Read the model definition and answer for the solid it produces. Units are mm, in the model's axes. Give positions to 0.01 mm unless a question says otherwise; leave off trailing zeros. Write each loop counter-clockwise with the first axis right and the second up, starting at its lowest first coordinate (ties: lowest second). Pieces come first, ordered by that corner, then holes. Notation, with made-up numbers: M 76.5,-9.75 L 107.5,-9.75 A19 cw 107.5,11.25 Z; hole C 17.5,42.5 d5. An arc over 180 degrees is marked long. Put each result on its own line as item: value.
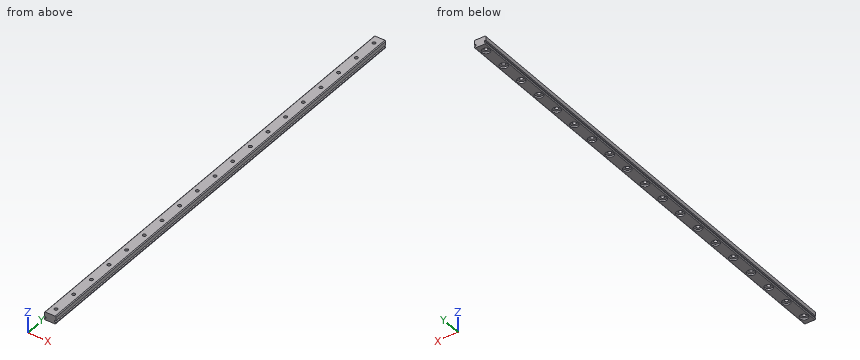
from build123d import *

# Parameters (mm, degrees)
EXTRUDE_1_DEPTH     = 280
SKETCH_2_R          = 1
CUT_EXTRUDE_1_DEPTH = 10
CHAMFER_1_SIZE      = 0.5
SKETCH_3_R          = 2.383304988
CUT_EXTRUDE_2_DEPTH = 1


with BuildPart() as part:
    # 草图1 → 凸台-拉伸1 (new body)
    with BuildSketch(Plane(origin=(0, 0, 0), x_dir=(1, 0, 0), z_dir=(0, 1, 0))):
        Polygon((-3.5, 0.4), (-3.5, -2.4), (3.5, -2.4), (3.5, 0.4), (2.5, 0.4), (2.5, 1.4), (3.5, 1.4), (3.5, 2.4), (-3.5, 2.4), (-3.5, 1.4), (-2.5, 1.4), (-2.5, 0.4), align=None)
    extrude(amount=EXTRUDE_1_DEPTH)

    # 草图2 → 切除-拉伸1 (cut)
    with BuildSketch(Plane(origin=(0, 0, -2.4), x_dir=(-1, 0, 0), z_dir=(0, 0, -1))):
        with Locations((0, 5)):
            Circle(SKETCH_2_R)
        with Locations((0, 20)):
            Circle(SKETCH_2_R)
        with Locations((0, 35)):
            Circle(SKETCH_2_R)
        with Locations((0, 50)):
            Circle(SKETCH_2_R)
        with Locations((0, 65)):
            Circle(SKETCH_2_R)
        with Locations((0, 80)):
            Circle(SKETCH_2_R)
        with Locations((0, 95)):
            Circle(SKETCH_2_R)
        with Locations((0, 110)):
            Circle(SKETCH_2_R)
        with Locations((0, 125)):
            Circle(SKETCH_2_R)
        with Locations((0, 140)):
            Circle(SKETCH_2_R)
        with Locations((0, 155)):
            Circle(SKETCH_2_R)
        with Locations((0, 170)):
            Circle(SKETCH_2_R)
        with Locations((0, 185)):
            Circle(SKETCH_2_R)
        with Locations((0, 200)):
            Circle(SKETCH_2_R)
        with Locations((0, 215)):
            Circle(SKETCH_2_R)
        with Locations((0, 230)):
            Circle(SKETCH_2_R)
        with Locations((0, 245)):
            Circle(SKETCH_2_R)
        with Locations((0, 260)):
            Circle(SKETCH_2_R)
        with Locations((0, 275)):
            Circle(SKETCH_2_R)
    extrude(amount=-CUT_EXTRUDE_1_DEPTH, mode=Mode.SUBTRACT)

    # 倒角1
    chamfer_1_edges = [part.edges().sort_by_distance(p)[0] for p in [
        (-3.5, 140, -2.4),
        (3.5, 140, -2.4),
        (3.5, 140, 2.4),
        (-3.5, 140, 2.4),
    ]]
    chamfer(chamfer_1_edges, length=CHAMFER_1_SIZE)

    # 草图3 → 切除-拉伸2 (cut)
    with BuildSketch(Plane(origin=(0, 0, -2.4), x_dir=(-1, 0, 0), z_dir=(0, 0, -1))):
        with Locations((0, 5)):
            Circle(SKETCH_3_R)
        with Locations((0, 20)):
            Circle(SKETCH_3_R)
        with Locations((0, 35)):
            Circle(SKETCH_3_R)
        with Locations((0, 50)):
            Circle(SKETCH_3_R)
        with Locations((0, 65)):
            Circle(SKETCH_3_R)
        with Locations((0, 80)):
            Circle(SKETCH_3_R)
        with Locations((0, 95)):
            Circle(SKETCH_3_R)
        with Locations((0, 110)):
            Circle(SKETCH_3_R)
        with Locations((0, 125)):
            Circle(SKETCH_3_R)
        with Locations((0, 140)):
            Circle(SKETCH_3_R)
        with Locations((0, 155)):
            Circle(SKETCH_3_R)
        with Locations((0, 170)):
            Circle(SKETCH_3_R)
        with Locations((0, 185)):
            Circle(SKETCH_3_R)
        with Locations((0, 200)):
            Circle(SKETCH_3_R)
        with Locations((0, 215)):
            Circle(SKETCH_3_R)
        with Locations((0, 230)):
            Circle(SKETCH_3_R)
        with Locations((0, 245)):
            Circle(SKETCH_3_R)
        with Locations((0, 260)):
            Circle(SKETCH_3_R)
        with Locations((0, 275)):
            Circle(SKETCH_3_R)
    extrude(amount=-CUT_EXTRUDE_2_DEPTH, mode=Mode.SUBTRACT)


solid = part.part
(1) Section A-A on z = 1.05 is taken. Give the number of separate pieces and of enclosed holes in the cut face, and give its area (3 significant figures).
Result:
separate pieces: 1
enclosed holes: 19
area: 1,900 mm²
(2) Given pin 1 Ø1.4 at (x, y) = (1, 276) entering from -Z; pin 2 Ø1.2 at (x, y) = (0, 275) entering from +Z, each flat-ended and moving along its own axis, determine where each tip first touches the part or whether it passes through.
Result:
pin 1: stops at z = -1.4
pin 2: passes through
(3) Straight lines are drawn through the part: line 1 along Z through (x, y) = (-2.75, 249.5); line 2 along X through (y, z) = (200, -1.8); line 3 along X through (y, z) = (200, 1.35). For each, find the intervals that lie inside material, in ascending order. Write a range as from..to.
Result:
line 1: z = -2.4..-1.4, -0.4..2.4
line 2: x = -3.5..-2.38, 2.38..3.5
line 3: x = -3.5..-1, 1..3.5
(4) Section B-B on y = 195 is taken. Determine the outline of the cut face in (x, z).
Result:
outline: M -3.5,-1.9 L -3,-2.4 L 3,-2.4 L 3.5,-1.9 L 3.5,-1.4 L 2.5,-1.4 L 2.5,-0.4 L 3.5,-0.4 L 3.5,1.9 L 3,2.4 L -3,2.4 L -3.5,1.9 L -3.5,-0.4 L -2.5,-0.4 L -2.5,-1.4 L -3.5,-1.4 Z
